```python
from build123d import *

# Parameters (mm, degrees)
ESBO_O1_W                = 50.1
ESBO_O1_H                = 48.1
ESBO_O1_W_2              = 42.05
ESBO_O1_H_2              = 40.05
RESSALTO_EXTRUS_O1_DEPTH = 20
ESBO_O3_W                = 50.1
ESBO_O3_H                = 48.1
RESSALTO_EXTRUS_O3_DEPTH = 4
ESBO_O4_R                = 11
CORTE_EXTRUS_O1_DEPTH    = 14
FILETE2_R                = 5


with BuildPart() as part:
    # Esboço1 → Ressalto-extrusão1 (new body)
    with BuildSketch(Plane.XY):
        with Locations((-2.099570717, -8.213533835)):
            Rectangle(ESBO_O1_W, ESBO_O1_H)
        with Locations((-2.124570717, -8.188533835)):
            Rectangle(ESBO_O1_W_2, ESBO_O1_H_2, mode=Mode.SUBTRACT)
    extrude(amount=RESSALTO_EXTRUS_O1_DEPTH)

    # Esboço3 → Ressalto-extrusão3 (add)
    with BuildSketch(Plane(origin=(0, 0, 0), x_dir=(-1, 0, 0), z_dir=(0, 0, -1))):
        with Locations((2.099570717, -8.213533835)):
            Rectangle(ESBO_O3_W, ESBO_O3_H)
    extrude(amount=RESSALTO_EXTRUS_O3_DEPTH)

    # Esboço4 → Corte-extrusão1 (cut)
    with BuildSketch(Plane.XZ.offset(32.263533835)):
        with Locations((-2.049570717, 21.15)):
            Circle(ESBO_O4_R)
    extrude(amount=-CORTE_EXTRUS_O1_DEPTH, mode=Mode.SUBTRACT)

    # Filete2
    filete2_edges = [part.edges().sort_by_distance(p)[0] for p in [
        (-27.149570717, 15.836466165, 8),
        (22.950429283, 15.836466165, 8),
        (22.950429283, -32.263533835, 8),
        (-27.149570717, -32.263533835, 8),
    ]]
    fillet(filete2_edges, radius=FILETE2_R)


solid = part.part
```
Can you work these out from the model? Positions are in its coordinate system, mm. A direction names the side the tool comes from. Give positions to 0.01 mm unless a question says otherwise; leave off trailing zeros. Order: outer loops, then holes, each group sorted by start corner. A loop starts at its lowest first (then second) coordinate and runs counter-clockwise, first axis right, second up. Notation, with made-up numbers: M -19.5,-22.75 L -10.5,-22.75 A29 ccw -10.5,-2.75 Z; hole C 42,-7.5 d9. An arc over 180 degrees is marked long. One line per item, written item: value.
1) We'd pull the mould along Y, two halves only. Please class faces 3 (the face through (-23.15, -8, 10)), 4 (the face through (-2.275, -30.267, 10.152)), 5 (the face through (-2, 15.836, 8)), 6 (the face through (-2, 11.836, 10)): released by +Y, released by -Y, zero draft, split by the parting line, or undercut.
Answer sheet:
face 3: undercut
face 4: zero draft
face 5: released by +Y
face 6: undercut
2) On a 3-axis mill with a long thin cutter (end or side, diameter ignored), from which of +Z, -Z, +X, -X, +Y, -Y can I reach the whole of each face in a straight line? I mean faces 1 (the face through (18.9, -8, 10)), 2 (the face through (-2, 15, 20)). Say none if no direction works.
Answer sheet:
face 1: +Z
face 2: +Z, +X, -X, +Y, -Y
3) I want a section at C-C, the plane z = 16. List the corners of the cut face in (x, y) for me, plus the area to 3 significant figures.
Answer sheet:
outline: M -27.15,-27.26 A5 ccw -22.15,-32.26 L -11.77,-32.26 L -11.77,-28.21 L -23.15,-28.21 L -23.15,11.84 L 18.9,11.84 L 18.9,-28.21 L 7.67,-28.21 L 7.67,-32.26 L 17.95,-32.26 A5 ccw 22.95,-27.26 L 22.95,10.84 A5 ccw 17.95,15.84 L -22.15,15.84 A5 ccw -27.15,10.84 Z
area: 626 mm^2
4) For P1, Ø10, axis at x = 13.5, y = -4, coming from the +Z side, with a flat end and sliding along its axis, tell me the tip position at first contact or that it passes through.
Answer sheet:
P1: stops at z = 0
5) I want a section at B-B, the plane z = 3.75. List the corners of the cut face in (x, y) for me, plus the area to 3 significant figures.
Answer sheet:
outline: M -27.15,-27.26 A5 ccw -22.15,-32.26 L 17.95,-32.26 A5 ccw 22.95,-27.26 L 22.95,10.84 A5 ccw 17.95,15.84 L -22.15,15.84 A5 ccw -27.15,10.84 Z; hole M -23.15,-28.21 L 18.9,-28.21 L 18.9,11.84 L -23.15,11.84 Z
area: 704 mm^2
6) Please list where these lines run through material, in increasing order: line 1 along X through (y, z) = (-18, 7); line 2 along Y through (x, z) = (-8, 8.25); line 3 along Z through (x, y) = (7, 7).
Answer sheet:
line 1: x = -27.15 to -23.15, 18.9 to 22.95
line 2: y = -32.26 to -28.21, 11.84 to 15.84
line 3: z = -4 to 0
7) I want a section at A-A, the plane y = -5.5. List the corners of the cut face in (x, z) for me, plus the area to 3 significant figures.
Answer sheet:
outline: M -27.15,-4 L 22.95,-4 L 22.95,20 L 18.9,20 L 18.9,0 L -23.15,0 L -23.15,20 L -27.15,20 Z
area: 361 mm^2
8) I want a section at D-D, the plane x = 1.5. List the corners of the cut face in (y, z) for me, plus the area to 3 significant figures.
Answer sheet:
outline: M -32.26,-4 L 15.84,-4 L 15.84,20 L 11.84,20 L 11.84,0 L -28.21,0 L -28.21,10.74 L -32.26,10.74 Z
area: 316 mm^2
